Input: dimensioned drawing with shaded views. Units: mm. Origin: part minimum x, y, z. A direction names the side the tool comes from. Give positions to 0.01 mm unless a question says otherwise; leave off trailing zeros. Write each loop counter-clockwise with the first axis right and the second up, starting at its lowest first coordinate (ties: lowest second). Pieces come first, ordered by that corner, then holes. Notation, with made-up numbers: (78.25, -6.5) -> (118.25, -6.5) arc R21 ccw to (118.25, 21.5) -> close; hole circle Ø2 at (83, 67.25). An arc over 180 degrees is marked (long way). Answer as a JSON object with one key per item and string values. Group by question number.
(1) Set-up query: the marked faces 4 and 5. Return all of +Z, -Z, +X, -X, +Y, -Y with unobstructed straight access to the full face (end or side cutting, diameter ignored); none if empty.
(2) Contact query for a flat-ended pin moving along its axis: pin 1 Ø4 at (x, y) = (10, 7) entering from +Z. Output: stop coordinate, or through.
(3) Material intervals for probe 1 along X at (y, z) = (9, 0.8); probe 2 along X at (y, z) = (3, 14.75), sorted ascending.
(4) Section query D-D on y = 12.25. Output: boundary loops of the cut face in (x, z), plus the area to 3 significant figures.
(5) Section query C-C on z = 8.25. Output: boundary loops of the cut face in (x, y).
(6) Section query A-A on y = 4. Output: boundary loops of the cut face in (x, z).
(7) Draft query along Y for the marked faces 1, 2 and 3. Return one class per face: +Y half, -Y half, draft (parallel to the pull), parting line (faces both ways), or undercut.
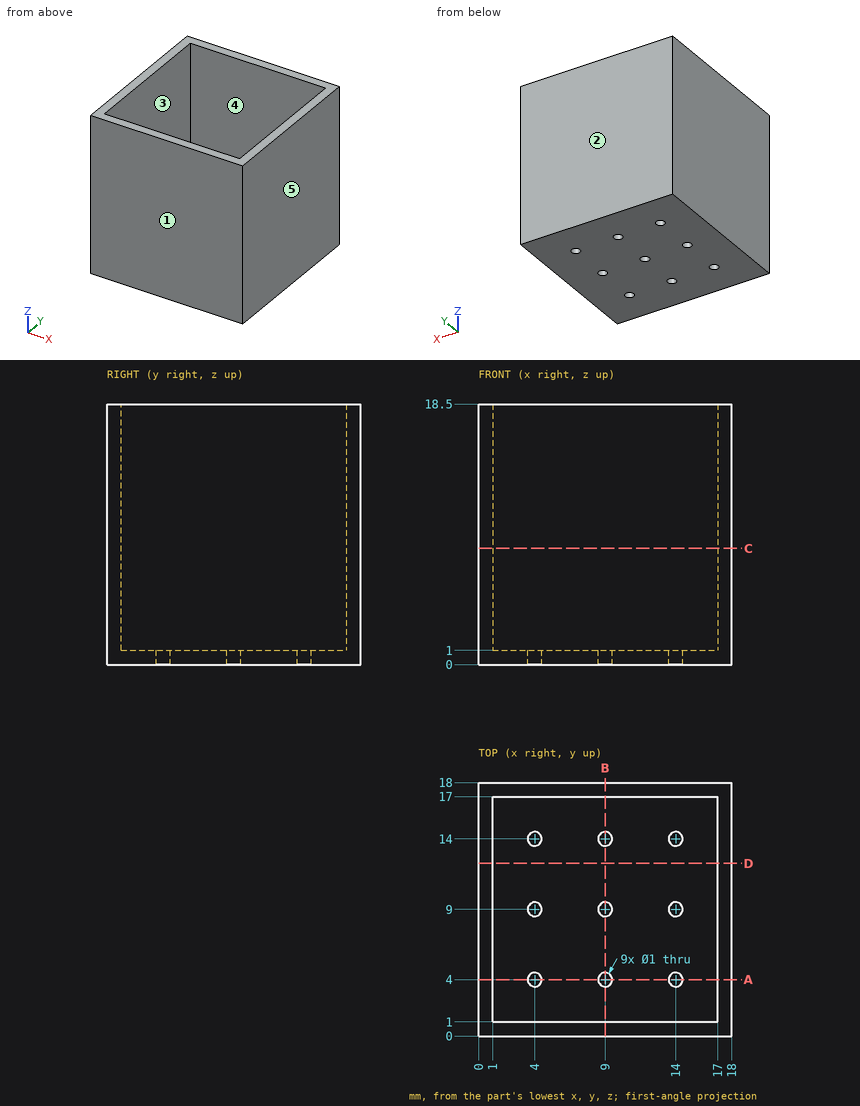
Answer list:
{
 "1": {"face 4": "+Z", "face 5": "+Z, -Z, +X, +Y, -Y"},
 "2": {"pin 1": "z = 1"},
 "3": {"probe 1": "0 to 3.5, 4.5 to 8.5, 9.5 to 13.5, 14.5 to 18", "probe 2": "0 to 1, 17 to 18"},
 "4": {"outline": "(0, 0) -> (18, 0) -> (18, 18.5) -> (17, 18.5) -> (17, 1) -> (1, 1) -> (1, 18.5) -> (0, 18.5) -> close", "area": "53.0 mm2"},
 "5": {"outline": "(0, 0) -> (18, 0) -> (18, 18) -> (0, 18) -> close; hole (1, 1) -> (17, 1) -> (17, 17) -> (1, 17) -> close"},
 "6": {"outline": "(0, 0) -> (3.5, 0) -> (3.5, 1) -> (1, 1) -> (1, 18.5) -> (0, 18.5) -> close; (4.5, 0) -> (8.5, 0) -> (8.5, 1) -> (4.5, 1) -> close; (9.5, 0) -> (13.5, 0) -> (13.5, 1) -> (9.5, 1) -> close; (14.5, 0) -> (18, 0) -> (18, 18.5) -> (17, 18.5) -> (17, 1) -> (14.5, 1) -> close"},
 "7": {"face 1": "-Y half", "face 2": "+Y half", "face 3": "undercut"}
}
